```python
from build123d import *

# Parameters (mm, degrees)
SKETCH2_R                     = 1.575
BOSS_EXTRUDE1_DEPTH           = 2.54
SKETCH3_R                     = 3.175
SKETCH3_R_2                   = 1.575
BOSS_EXTRUDE2_DEPTH           = 0.635
SKETCH4_W                     = 6.35
SKETCH4_H                     = 3
BOSS_EXTRUDE3_DEPTH           = 1
SKETCH5_W                     = 6.35
SKETCH5_H                     = 3
BOSS_EXTRUDE4_DEPTH           = 2
BOSS_EXTRUDE4_DRAFT           = 3
BOSS_EXTRUDE4_PROFILE_2_DEPTH = 2
BOSS_EXTRUDE4_PROFILE_2_DRAFT = 3
SKETCH6_R                     = 1.55
CUT_EXTRUDE1_DEPTH            = 19.05
CUT_EXTRUDE2_START            = -0.788
SKETCH7_W                     = 3.1
SKETCH7_H                     = 6.35
SKETCH7_H_2                   = 4.7625
CUT_EXTRUDE2_DEPTH            = 0.788
CUT_EXTRUDE3_REACH            = 195.613
SKETCH8_W                     = 1.27
SKETCH8_H                     = 6.35
LPATTERN1_COUNT               = 2
LPATTERN1_PITCH               = 25.4


with BuildPart() as part:
    # Sketch2 → Boss-Extrude1 (new body)
    with BuildSketch(Plane.XY):
        with BuildLine():
            Line((186.055, 33.49625), (189.23, 31.115))
            ThreePointArc((189.23, 31.115), (190.164806331, 29.994903166), (190.5, 28.575))
            Line((190.5, 28.575), (190.5, 0))
            Line((190.5, 0), (154.305, 0))
            Line((154.305, 0), (154.305, 29.44))
            ThreePointArc((154.305, 29.44), (154.676974388, 30.338025612), (155.575, 30.71))
            Line((155.575, 30.71), (161.925, 30.71))
            ThreePointArc((161.925, 30.71), (162.482139282, 30.58126939), (162.926332297, 30.221174521))
            Line((162.926332297, 30.221174521), (166.306150062, 25.888825479))
            ThreePointArc((166.306150062, 25.888825479), (166.750343077, 25.52873061), (167.307482358, 25.4))
            Line((167.307482358, 25.4), (175.563715168, 25.4))
            ThreePointArc((175.563715168, 25.4), (176.141475824, 25.539030228), (176.592738534, 25.925680906))
            Line((176.592738534, 25.925680906), (181.577441586, 32.817047734))
            ThreePointArc((181.577441586, 32.817047734), (183.673830399, 34.095340236), (186.055, 33.49625))
        make_face()
        with Locations((184.15, 30.95625)):
            Circle(SKETCH2_R, mode=Mode.SUBTRACT)
    extrude(amount=BOSS_EXTRUDE1_DEPTH)

    # Sketch3 → Boss-Extrude2 (add)
    with BuildSketch(Plane.XY.offset(2.54)):
        with Locations(Location((184.15, 30.95625, 0), (0, 0, 144.120815799))):
            Circle(SKETCH3_R)
        with Locations((184.15, 30.95625)):
            Circle(SKETCH3_R_2, mode=Mode.SUBTRACT)
    extrude(amount=BOSS_EXTRUDE2_DEPTH)

    # Sketch4 → Boss-Extrude3 (add)
    with BuildSketch(Plane(origin=(0, 0, 0), x_dir=(-1, 0, 0), z_dir=(0, 0, -1))):
        with Locations((-184.15, 27.94)):
            Rectangle(SKETCH4_W, SKETCH4_H)
        with Locations((-158.75, 27.94)):
            Rectangle(SKETCH4_W, SKETCH4_H)
    extrude(amount=BOSS_EXTRUDE3_DEPTH)


with BuildPart() as boss_extrude4_tool:
    # Sketch5 → Boss-Extrude4 (with draft: the straight prism first)
    with BuildSketch(Plane(origin=(0, 0, -1), x_dir=(-1, 0, 0), z_dir=(0, 0, -1))):
        with Locations((-158.75, 27.94)):
            Rectangle(SKETCH5_W, SKETCH5_H)
    extrude(amount=BOSS_EXTRUDE4_DEPTH)
    # Boss-Extrude4: the draft: its side faces are tilted about the plane it starts from
    boss_extrude4_sides = [boss_extrude4_tool.faces().sort_by_distance(p)[0] for p in [
        (155.575, 27.94, -2),
        (158.75, 29.44, -2),
        (161.925, 27.94, -2),
        (158.75, 26.44, -2),
    ]]
    draft(boss_extrude4_sides, Plane(origin=(0, 0, -1), x_dir=(-1, 0, 0), z_dir=(0, 0, -1)), BOSS_EXTRUDE4_DRAFT)


with BuildPart() as part_1:
    add(part.part)

    # Boss-Extrude4: add boss_extrude4_tool
    add(boss_extrude4_tool.part)


with BuildPart() as boss_extrude4_profile_2_tool:
    # Sketch5 → Boss-Extrude4 profile 2 (with draft: the straight prism first)
    with BuildSketch(Plane(origin=(0, 0, -1), x_dir=(-1, 0, 0), z_dir=(0, 0, -1))):
        with Locations((-184.15, 27.94)):
            Rectangle(SKETCH5_W, SKETCH5_H)
    extrude(amount=BOSS_EXTRUDE4_PROFILE_2_DEPTH)
    # Boss-Extrude4 profile 2: the draft: its side faces are tilted about the plane it starts from
    boss_extrude4_profile_2_sides = [boss_extrude4_profile_2_tool.faces().sort_by_distance(p)[0] for p in [
        (180.975, 27.94, -2),
        (184.15, 29.44, -2),
        (187.325, 27.94, -2),
        (184.15, 26.44, -2),
    ]]
    draft(boss_extrude4_profile_2_sides, Plane(origin=(0, 0, -1), x_dir=(-1, 0, 0), z_dir=(0, 0, -1)), BOSS_EXTRUDE4_PROFILE_2_DRAFT)


with BuildPart() as part_2:
    add(part_1.part)

    # Boss-Extrude4 profile 2: add boss_extrude4_profile_2_tool
    add(boss_extrude4_profile_2_tool.part)

    # Sketch6 → Cut-Extrude1 (cut)
    with BuildSketch(Plane.XZ):
        with Locations((184.15, 1.752)):
            Circle(SKETCH6_R)
    cut_extrude1 = extrude(amount=-CUT_EXTRUDE1_DEPTH, mode=Mode.SUBTRACT)

    # Sketch7 → Cut-Extrude2 (cut)
    with BuildSketch(Plane.XY.offset(2.54).offset(CUT_EXTRUDE2_START)):
        with Locations((184.15, 15.875)):
            Rectangle(SKETCH7_W, SKETCH7_H)
        with Locations((184.15, 2.38125)):
            Rectangle(SKETCH7_W, SKETCH7_H_2)
    cut_extrude2 = extrude(amount=CUT_EXTRUDE2_DEPTH, mode=Mode.SUBTRACT)

    # Sketch8 → Cut-Extrude3 (cut, up to next)
    with BuildSketch(Plane.XY.offset(2.54), mode=Mode.PRIVATE) as cut_extrude3_sk1:
        with Locations((184.15, 3.175)):
            Rectangle(SKETCH8_W, SKETCH8_H)
    cut_extrude3_tool1 = extrude(cut_extrude3_sk1.sketch, amount=-CUT_EXTRUDE3_REACH, mode=Mode.PRIVATE) & part_2.part
    cut_extrude3 = cut_extrude3_tool1.solids().sort_by_distance((184.15, 3.175, 2.54))[0]
    add(cut_extrude3, mode=Mode.SUBTRACT)

    # LPattern1: Cut-Extrude1, Cut-Extrude2, Cut-Extrude3 ×2
    with Locations(*[(-i * LPATTERN1_PITCH, 0, 0) for i in range(1, LPATTERN1_COUNT)]):
        add(cut_extrude1, mode=Mode.SUBTRACT)
        add(cut_extrude2, mode=Mode.SUBTRACT)
        add(cut_extrude3, mode=Mode.SUBTRACT)

    # Mirror1: part across plane


with BuildPart() as part_3:
    add(part_2.part)
    add(part_2.part.mirror(Plane.ZX))


solid = part_3.part
```
Part model, mm, in its own coordinate system. A direction names the side the tool comes from. Round coordinates to 2 decimals unless told otherwise and drop trailing zeros. Loops run counter-clockwise (first coordinate to the right, second up) from the corner with the lowest first, then second, coordinate; pieces in that order, holes last.
1. Slice it at B-B (x = 158.75). Give the cut face in (y, z).
Solutions:
outline: (-30.71, 0) - (-29.44, 0) - (-29.44, -1) - (-29.34, -3) - (-26.54, -3) - (-26.44, -1) - (-26.44, 0) - (-6.35, 0) - (-6.35, 0.2) - (-19.05, 0.2) - (-19.05, 2.54) - (-30.71, 2.54) - close; (6.35, 0) - (26.44, 0) - (26.44, -1) - (26.54, -3) - (29.34, -3) - (29.44, -1) - (29.44, 0) - (30.71, 0) - (30.71, 2.54) - (19.05, 2.54) - (19.05, 0.2) - (6.35, 0.2) - close
2. Two-plate mould, pull along X, no slides. Class faces 1 (the face through (185.37, 0.267, 0.795)), 2 (the face through (184.19, 29.39, -1.99)), 3 (the face through (154.67, 30.33, 1.25)), 4 (the face through (187.62, -32.322, 1.252)): pulls with the +X half, pulls with the -X half, needs draft (parallel to the pull), parting line crosses it, or undercut.
Solutions:
face 1: undercut
face 2: needs draft
face 3: pulls with the -X half
face 4: pulls with the +X half
3. Drill centre lines: line 1 along Y through (x, z) = (184.15, 1.2); line 2 along Y through (x, z) = (183, 1); line 3 along X through (y, z) = (-14.5, 2) (3 decimals). Where is each one in solid material? Low to high.
Solutions:
line 1: y = -34.13 to -32.53, -29.38 to -19.05, 19.05 to 29.38, 32.53 to 34.13
line 2: y = -33.92 to -32.03, -29.88 to -19.05, 19.05 to 29.88, 32.03 to 33.92
line 3: x = 154.305 to 157.2, 160.3 to 182.6, 185.7 to 190.5
4. 3-axis set-ups, long thin cutter, end or side, ignore diameter. For faces 5 (the face through (184.19, -26.49, -1.99)), 6 (the face through (184, 19.05, 2)), 7 (the face through (159, -30.71, 1)), 8 (the face through (159, 30.71, 1)): which of +Z, -Z, +X, -X, +Y, -Y reach the whole face in a straight line?
Solutions:
face 5: -Z, +X, -X
face 6: +Z
face 7: +Z, -Z, -X, -Y
face 8: +Z, -Z, -X, +Y
5. Slice it at D-D (x = 165.5). Give the cut face in (y, z).
Solutions:
outline: (-26.92, 0) - (26.92, 0) - (26.92, 2.54) - (-26.92, 2.54) - close
6. Slice it at A-A (y = 1). Give the cut face in (x, z) (3 decimals), and give its area (3 significant figures).
Solutions:
outline: (154.305, 0) - (158.115, 0) - (158.115, 0.338) arc R1.55 cw to (157.2, 1.752) - (157.2, 2.54) - (154.305, 2.54) - close; (159.385, 0) - (183.515, 0) - (183.515, 0.338) arc R1.55 cw to (182.6, 1.752) - (182.6, 2.54) - (160.3, 2.54) - (160.3, 1.752) arc R1.55 cw to (159.385, 0.338) - close; (184.785, 0) - (190.5, 0) - (190.5, 2.54) - (185.7, 2.54) - (185.7, 1.752) arc R1.55 cw to (184.785, 0.338) - close
area: 78.9 mm2
7. Flat gauge pins, fed straight in: pin 1 (12 mm diameter, centred on x = 172, y = -20, fed in from -Z); pin 2 (1.5 mm diameter, centred on y = 18.5, z = -2, fed in from +X); pin 3 (5 mm diameter, centred on x = 164, y = -4, fed in from +Z); pin 4 (3 mm diameter, centred on x = 178, z = 2, fed in from +Y) (3 decimals). Where does each tip first touch, or does it go through?
Solutions:
pin 1: stops at z = 0
pin 2: passes through
pin 3: stops at z = 2.54
pin 4: stops at y = 29.945
8. Slice it at C-C (y = -18). Give the cut face in (x, z) (3 decimals), and give its area (3 significant figures).
Solutions:
outline: (154.305, 0) - (190.5, 0) - (190.5, 2.54) - (185.7, 2.54) - (185.7, 1.752) arc R1.55 cw to (182.6, 1.752) - (182.6, 2.54) - (160.3, 2.54) - (160.3, 1.752) arc R1.55 cw to (157.2, 1.752) - (157.2, 2.54) - (154.305, 2.54) - close
area: 79.5 mm2
